For this review, take the finished solid that the model builds, in its own axes (mm). Face numbers are marked on the shaded views. A direction names the side the tool comes from. Give positions to 0.01 mm unless a question says otherwise; leave off trailing zeros. Order: outer loops, then holes, each group sorted by start corner. A loop starts at its lowest first (then second) coordinate and runs counter-clockwise, first axis right, second up. Notation, with made-up numbers: (21, -25) - (48, -25) arc R22 ccw to (48, 7) - close; hole circle Ø8 at (31, 38.5). An arc over 180 degrees is marked (long way). Answer as a JSON object with one key per item and string values. Group by question number.
from build123d import *

# Parameters (mm, degrees)
SKETCH1_R           = 15
BOSS_EXTRUDE2_DEPTH = 194
SKETCH2_W           = 50.475671087
SKETCH2_H           = 50.915354634
BOSS_EXTRUDE3_DEPTH = 34
SKETCH3_R           = 7.5
BOSS_EXTRUDE4_DEPTH = 99
SKETCH5_R           = 42.253100096
BOSS_EXTRUDE5_DEPTH = 10


with BuildPart() as part:
    # Sketch1 → Boss-Extrude2 (new body)
    with BuildSketch(Plane(origin=(0, 0, 0), x_dir=(1, 0, 0), z_dir=(0, 1, 0))):
        with Locations(Location((0, 0, 0), (0, 0, 270))):
            Circle(SKETCH1_R)
    extrude(amount=BOSS_EXTRUDE2_DEPTH)

    # Sketch2 → Boss-Extrude3 (add)
    with BuildSketch(Plane.XZ):
        with Locations((0.175873419, 0)):
            Rectangle(SKETCH2_W, SKETCH2_H)
    boss_extrude3 = extrude(amount=BOSS_EXTRUDE3_DEPTH)

    # Mirror1: Boss-Extrude3 across plane
    add(boss_extrude3.mirror(Plane.ZX.offset(90)))

    # Sketch3 → Boss-Extrude4 (add)
    with BuildSketch(Plane.XZ.offset(34)):
        with Locations(Location((0, 0, 0), (0, 0, 90))):
            Circle(SKETCH3_R)
    extrude(amount=BOSS_EXTRUDE4_DEPTH)

    # Sketch5 → Boss-Extrude5 (add)
    with BuildSketch(Plane.XZ.offset(133)):
        with Locations(Location((0, 0, 0), (0, 0, 270))):
            Circle(SKETCH5_R)
    extrude(amount=BOSS_EXTRUDE5_DEPTH)


solid = part.part
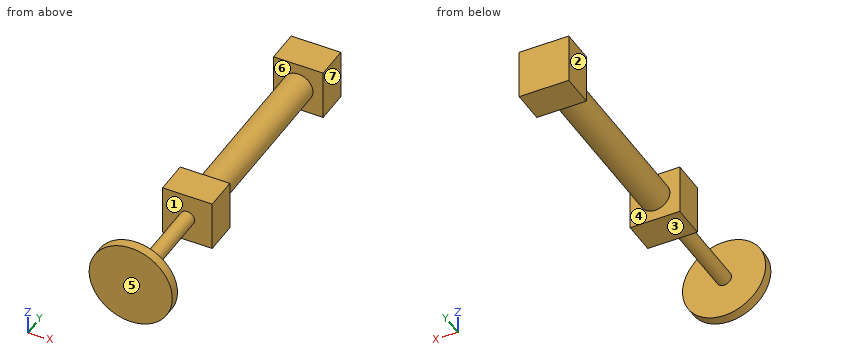
1) For line 1 (Y direction, x = 15, z = -7); line 2 (Y direction, x = 12, z = -2); line 3 (Y direction, x = -4, z = -32), list the stretches that pass through material, from the lowest coordinate up.
2) Consider section C-C (y = -48.5). Give the boundary of the cut face in (x, z).
3) For pin 1 (10 mm diameter, centred on x = -30, z = -31.5, fed in from +Y); pin 2 (10 mm diameter, centred on x = 2.5, y = -25.5, fed in from +Z); pin 3 (10 mm diameter, centred on y = -21.5, z = -2, fed in from -X), all flat-tipped, find the tip position at first contact; note any pin that passes through.
4) Consider section B-B (z = 0). Give the boundary of the cut face in (x, y), plus the area to 3 significant figures.
5) Mouldability with a two-part tool opening along Y and no side actions: class the marked faces 4, 5, 6 and 7 as released by +Y, released by -Y, zero draft, split by the parting line, or undercut.
6) Consider section A-A (x = 0). Give the boundary of the cut face in (y, z), plus the area to 3 significant figures.
7) For the marked faces 1, 2 and 3, list the 3-axis set-ups (+Z, -Z, +X, -X, +Y, -Y) from which the entire face can be reached by the end or side of a thin tool; tool diameter is ignored.
8) Consider section D-D (y = 20.5). Give the boundary of the cut face in (x, z), plus the area to 3 significant figures.
Result set:
{
 "1": {"line 1": "y = -143 to -133, -34 to 0, 180 to 214", "line 2": "y = -143 to -133, -34 to 214", "line 3": "y = -143 to -133"},
 "2": {"outline": "circle Ø15 at (0, 0)"},
 "3": {"pin 1": "stops at y = -133", "pin 2": "stops at z = 25.46", "pin 3": "stops at x = -25.06"},
 "4": {"outline": "(-42.25, -143) - (42.25, -143) - (42.25, -133) - (7.5, -133) - (7.5, -34) - (25.41, -34) - (25.41, 0) - (15, 0) - (15, 180) - (25.41, 180) - (25.41, 214) - (-25.06, 214) - (-25.06, 180) - (-15, 180) - (-15, 0) - (-25.06, 0) - (-25.06, -34) - (-7.5, -34) - (-7.5, -133) - (-42.25, -133) - close", "area": "11,200 mm2"},
 "5": {"face 4": "undercut", "face 5": "released by -Y", "face 6": "undercut", "face 7": "zero draft"},
 "6": {"outline": "(-143, -42.25) - (-133, -42.25) - (-133, -7.5) - (-34, -7.5) - (-34, -25.46) - (0, -25.46) - (0, -15) - (180, -15) - (180, -25.46) - (214, -25.46) - (214, 25.46) - (180, 25.46) - (180, 15) - (0, 15) - (0, 25.46) - (-34, 25.46) - (-34, 7.5) - (-133, 7.5) - (-133, 42.25) - (-143, 42.25) - close", "area": "11,200 mm2"},
 "7": {"face 1": "none", "face 2": "+Z, -Z, -X, +Y", "face 3": "-Z, +X, -X, +Y"},
 "8": {"outline": "circle Ø30 at (0, 0)", "area": "707 mm2"}
}
